Solid Edge part; units mm, degrees
sketch "Sketch1" plane through (0, 0, 0) normal (0, -1, 0) x (1, 0, 0)
  line L0 (80, 35) -> (80, 0)
  line L1 (80, 0) -> (0, 0)
  line L2 (0, 0) -> (0, 65)
  line L3 (0, 65) -> (45, 65)
  line L4 (45, 65) -> (45, 35)
  line L5 (45, 35) -> (80, 35)
extrude "ExtrudedProtrusion_1" add sketch "Sketch1" along normal mid plane 70
sketch "Sketch2" plane through (45, 0, 50) normal (1, 0, 0) x (0, 1, 0)
  line L0 (-35, 15) -> (-35, -15)
  line L1 (-35, -15) -> (-3, 15)
  line L2 (-3, 15) -> (-35, 15)
extrude "ExtrudedCutout_1" cut sketch "Sketch2" against normal blind 20
sketch "Sketch3" plane through (80, 0, 35) normal (0.5774, -0.5774, 0.5774) x (-0.7071, -0.7071, 0)
  line L0 (24.7487, 42.8661) -> (0, 0)
  line L1 (0, 0) -> (49.4975, 0)
  line L2 (49.4975, 0) -> (24.7487, 42.8661)
extrude "Cutout1" cut sketch "Sketch3" along normal up to next
Design review of the part built by this model. Coordinates are the model's own, in mm. A direction names the side the tool comes from. Coordinates: 2 decimals unless noted, no trailing zeros. Order: outer loops, then holes, each group sorted by start corner. A loop starts at its lowest first (then second) coordinate and runs counter-clockwise, first axis right, second up.
1) For faces 1 (the flat face through (25, -26, 56)), 2 (the flat face through (45, 8, 50)), 3 (the flat face through (17, 8, 65)), list the 3-axis set-ups (+Z, -Z, +X, -X, +Y, -Y) from which the entire face can be reached by the end or side of a thin tool; tool diameter is ignored.
2) Take a section at C-C, the plane y = 10. Give the boundary of the cut face in (x, z).
3) Take a section at A-A, the plane x = 63. Give the boundary of the cut face in (y, z), and give its area (3 significant figures).
4) Wall thickness on line 1 along X through (y, z) = (-20, 36.5); line 2 along Z through (x, y) = (51, 11.5); line 3 along Y through (x, z) = (72.5, 18.5): over which ranges is each line inside the solid? List them lowest first.
5) Take a section at B-B, the plane z = 38. Give the boundary of the cut face in (x, y), and give its area (3 significant figures).
6) Take a section at D-D, the plane x = 29. Give the boundary of the cut face in (y, z), and give its area (3 significant figures).
7) Clearance check with flat-ended pins moving along their axes: pin 1 (15 mm diameter, centred on y = 17.5, z = 52.5, fed in from +X); pin 2 (3 mm diameter, centred on x = 57, y = -18.5, fed in from +Z); pin 3 (9 mm diameter, centred on y = -22, z = 54.5, fed in from +X). State where each tip first meets the part, or that it passes through.
Returned:
1. face 1: +Z, +X, -Y
1. face 2: +Z, +X, +Y, -Y
1. face 3: +Z, +X, -X, +Y, -Y
2. outline: (0, 0) - (80, 0) - (80, 35) - (45, 35) - (45, 65) - (0, 65) - close
3. outline: (-35, 0) - (35, 0) - (35, 35) - (-17, 35) - (-35, 17) - close
3. area: 2,290 mm2
4. line 1: x = 0 to 45
4. line 2: z = 0 to 35
4. line 3: y = -24 to 35
5. outline: (0, -35) - (25, -35) - (25, -31.8) - (45, -31.8) - (45, 35) - (0, 35) - close
5. area: 3,090 mm2
6. outline: (-35, 0) - (35, 0) - (35, 65) - (-3, 65) - (-35, 35) - close
6. area: 4,070 mm2
7. pin 1: stops at x = 45
7. pin 2: stops at z = 35
7. pin 3: stops at x = 25
